Check sheet for the modelled part. Datum: model origin and axes. Units: mm. A direction names the side the tool comes from. Coordinates: 2 decimals unless noted, no trailing zeros. Loops run counter-clockwise (first coordinate to the right, second up) from the corner with the lowest first, then second, coordinate; pieces in that order, holes last.
```python
from build123d import *

# Parameters (mm, degrees)
F1_DEPTH  = 7.62
F3_W      = 0.635
F3_H      = 5.842
F6_DEPTH  = 12.7
F7_R      = 0.127
F9_W      = 10.16
F9_H      = 1.27
F10_DEPTH = 3.175


with BuildPart() as f1:
    # F0 (on Top) → F1 (new body)
    with BuildSketch(Plane.XY):
        with BuildLine():
            Line((10.9985226281, 0), (0.508, 0))
            ThreePointArc((0.508, 0), (0.1487897552, -0.1487897552), (0, -0.508))
            Line((0, -0.508), (0, -0.762))
            ThreePointArc((0, -0.762), (0.1487897552, -1.1212102448), (0.508, -1.27))
            Line((0.508, -1.27), (10.9985226281, -1.27))
            ThreePointArc((10.9985226281, -1.27), (12.3133233772, -1.4430968025), (13.5385226281, -1.9505909488))
            Line((13.5385226281, -1.9505909488), (21.7479125756, -6.6902844449))
            ThreePointArc((21.7479125756, -6.6902844449), (21.8610174728, -6.9931140452), (21.5852173248, -7.1617342188))
            Line((21.5852173248, -7.1617342188), (11.0182697374, -5.6618500829))
            ThreePointArc((11.0182697374, -5.6618500829), (10.6417144767, -5.7586825509), (10.4439205931, -6.093418224))
            Line((10.4439205931, -6.093418224), (10.4082253422, -6.3448975453))
            ThreePointArc((10.4082253422, -6.3448975453), (10.5050578102, -6.7214528061), (10.8397934833, -6.9192466897))
            Line((10.8397934833, -6.9192466897), (24.0516598784, -8.7945535034))
            ThreePointArc((24.0516598784, -8.7945535034), (25.144685653, -8.1262935433), (24.6964387295, -6.9261471298))
            Line((24.6964387295, -6.9261471298), (14.1735226281, -0.850738686))
            ThreePointArc((14.1735226281, -0.850738686), (12.6420235645, -0.2163710031), (10.9985226281, 0))
        make_face()
    extrude(amount=F1_DEPTH)

    # F3 (on offset) → F4 (revolve)
    with BuildSketch(Plane.XY.offset(3.81)):
        Polygon((3.81, 3.048), (3.81, 0), (5.842, 0), (5.842, 8.89), (4.445, 8.89), (4.445, 3.048), align=None)
        with BuildLine():
            Line((4.445, 8.89), (5.842, 8.89))
            Line((5.842, 8.89), (6.35, 8.89))
            ThreePointArc((6.35, 8.89), (5.8180463142, 10.4454259867), (4.445, 11.3493444248))
            Line((4.445, 11.3493444248), (4.445, 8.89))
        make_face()
        with BuildLine():
            Line((3.81, 11.43), (3.81, 8.89))
            Line((3.81, 8.89), (4.445, 8.89))
            Line((4.445, 8.89), (4.445, 11.3493444248))
            ThreePointArc((4.445, 11.3493444248), (4.1300509029, 11.4097554285), (3.81, 11.43))
        make_face()
        with Locations((4.1275, 5.969)):
            Rectangle(F3_W, F3_H)
    revolve(axis=Axis((3.81, 4.445, 3.81), (0, 1, 0)))

    # F5 (on offset) → F6 (cut, symmetric)
    with BuildSketch(Plane.XY.offset(3.81)):
        Polygon((3.175, 3.048), (3.81, 3.048), (4.445, 3.048), (4.445, 13.208), (3.175, 13.208), align=None)
    extrude(amount=F6_DEPTH, both=True, mode=Mode.SUBTRACT)

    # F7
    f7_edges = [f1.edges().sort_by_distance(p)[0] for p in [
        (1.27, 8.89, 3.81),
        (6.35, 8.89, 3.81),
    ]]
    fillet(f7_edges, radius=F7_R)

    # F9 (on offset) → F10 (cut, symmetric)
    with BuildSketch(Plane(origin=(3.81, 0, 0), x_dir=(0, -1, 0), z_dir=(-1, 0, 0))):
        with Locations((-8.128, 3.81)):
            Rectangle(F9_W, F9_H)
    extrude(amount=F10_DEPTH, both=True, mode=Mode.SUBTRACT)


solid = f1.part
```
1) Section check C-C on z = 3.81. Enter the section's corners in (x, y).
Answer sheet:
outline: (0, -0.76) arc R0.51 ccw to (0.51, -1.27) - (11, -1.27) arc R5.08 cw to (13.54, -1.95) - (21.75, -6.69) arc R0.25 cw to (21.59, -7.16) - (11.02, -5.66) arc R0.51 ccw to (10.44, -6.09) - (10.41, -6.34) arc R0.51 ccw to (10.84, -6.92) - (24.05, -8.79) arc R1.01 ccw to (24.7, -6.93) - (14.17, -0.85) arc R6.35 ccw to (11, 0) - (5.84, 0) - (5.84, 3.05) - (1.78, 3.05) - (1.78, 0) - (0.51, 0) arc R0.51 ccw to (0, -0.51) - close
2) Section check A-A on y = 6.5. Enter the section's corners in (x, z) (3 decimals), plus the area to 3 significant figures.
Answer sheet:
outline: (1.88, 3.175) arc R2.032 ccw to (3.175, 1.88) - (3.175, 3.175) - close; (1.88, 4.445) - (3.175, 4.445) - (3.175, 5.74) arc R2.032 ccw to start; (4.445, 1.88) arc R2.032 ccw to (5.74, 3.175) - (4.445, 3.175) - close; (4.445, 4.445) - (5.74, 4.445) arc R2.032 ccw to (4.445, 5.74) - close
area: 4.43 mm2
3) Mould release check, pull along Y, two halves, no side actions. Record for faces 4 (the flat face through (16.376, -6.422, 3.757)), 5 (the flat face through (2.27, 8.89, 2.26)), 6 (the flat face through (2.5, 7.2, 3.175)), 7 (the cylindrical face through (12.66, -0.22, 3.76)): +Y half, -Y half, draft (parallel to the pull), parting line (faces both ways), or undercut.
Answer sheet:
face 4: undercut
face 5: undercut
face 6: draft
face 7: +Y half
4) Section check D-D on x = 12.25. Enter the section's corners in (y, z), plus the area to 3 significant figures.
Answer sheet:
outline: (-7.12, 0) - (-5.84, 0) - (-5.84, 7.62) - (-7.12, 7.62) - close; (-1.43, 0) - (-0.12, 0) - (-0.12, 7.62) - (-1.43, 7.62) - close
area: 19.7 mm2
5) Set-up check for faces 1 (the flat face through (17.59, -4.29, 3.76)), 2 (the flat face through (5.4, 8.89, 2.3)), 3 (the flat face through (2.5, 7.2, 4.445)): record each of +Z, -Z, +X, -X, +Y, -Y from which the full face is reachable in a straight line by a thin tool's end or side.
Answer sheet:
face 1: +Z, -Z
face 2: -Z, +X
face 3: +X, -X, +Y
6) Depth check by flat-ended pin: pin 1 (1.4 mm diameter, centred on x = 2.5, z = 2.5, fed in from -Y); pin 2 (0.5 mm diameter, centred on y = 6, z = 2.5, fed in from -X); pin 3 (4 mm diameter, centred on y = 9, z = 3, fed in from +X). Enter the tip coordinate at first touch or a pass-through.
Answer sheet:
pin 1: stops at y = -1.27
pin 2: stops at x = 2.08
pin 3: stops at x = 6.27
7) Section check B-B on x = 3.81. Enter the section's corners in (y, z), plus the area to 3 significant figures.
Answer sheet:
outline: (-1.27, 0) - (0, 0) - (0, 1.78) - (3.05, 1.78) - (3.05, 5.84) - (0, 5.84) - (0, 7.62) - (-1.27, 7.62) - close
area: 22.1 mm2
8) Scan lines: line 1 (X direction, y = 8.5, z = 5) (3 decimals); line 2 (Y direction, x = 20.25, z = 3); line 3 (X direction, y = 9.75, z = 2) (3 decimals). Record each from-to range of solid material in increasing order.
Answer sheet:
line 1: x = 2.163 to 3.175, 4.445 to 5.457
line 2: y = -8.25 to -6.97, -5.83 to -4.36
line 3: x = 2.249 to 3.175, 4.445 to 5.371
